```python
from build123d import *

# Parameters (mm, degrees)
SKETCH_1_R          = 32
SKETCH_1_R_2        = 24
EXTRUDE_1_DEPTH     = 2
SKETCH_2_R          = 32
SKETCH_2_R_2        = 25
EXTRUDE_2_DEPTH     = 4
SKETCH_3_R          = 1.8
CUT_EXTRUDE_1_DEPTH = 46.650848842
CUT_EXTRUDE_2_DEPTH = 2.8
SKETCH_6_R          = 1.8
CUT_EXTRUDE_3_DEPTH = 46.367830012
CUT_EXTRUDE_4_DEPTH = 2.8
FILLET_1_R          = 1


with BuildPart() as part:
    # 草图1 → 凸台-拉伸1 (new body)
    with BuildSketch(Plane.XY):
        Circle(SKETCH_1_R)
        Circle(SKETCH_1_R_2, mode=Mode.SUBTRACT)
    extrude(amount=EXTRUDE_1_DEPTH)

    # 草图2 → 凸台-拉伸2 (add)
    with BuildSketch(Plane.XY.offset(2)):
        Circle(SKETCH_2_R)
        Circle(SKETCH_2_R_2, mode=Mode.SUBTRACT)
    extrude(amount=EXTRUDE_2_DEPTH)

    # 草图3 → 切除-拉伸1 (cut, through all)
    with BuildSketch(Plane.XY.offset(6)):
        with Locations((0, 28.5)):
            Circle(SKETCH_3_R)
        with Locations((24.681724008, 14.25)):
            Circle(SKETCH_3_R)
        with Locations((24.681724008, -14.25)):
            Circle(SKETCH_3_R)
        with Locations((0, -28.5)):
            Circle(SKETCH_3_R)
        with Locations((-24.681724008, -14.25)):
            Circle(SKETCH_3_R)
        with Locations((-24.681724008, 14.25)):
            Circle(SKETCH_3_R)
    extrude(amount=-CUT_EXTRUDE_1_DEPTH, mode=Mode.SUBTRACT)

    # 草图5 → 切除-拉伸2 (cut)
    with BuildSketch(Plane.XY.offset(6)):
        Polygon((-17.866352837, 22.43873369), (-20.989347038, 23.275537464), (-23.275537464, 20.989347038), (-22.43873369, 17.866352837), (-19.31573949, 17.029549063), (-17.029549063, 19.31573949), align=None)
        Polygon((22.43873369, 17.866352837), (23.275537464, 20.989347038), (20.989347038, 23.275537464), (17.866352837, 22.43873369), (17.029549063, 19.31573949), (19.31573949, 17.029549063), align=None)
        Polygon((17.866352837, -22.43873369), (20.989347038, -23.275537464), (23.275537464, -20.989347038), (22.43873369, -17.866352837), (19.31573949, -17.029549063), (17.029549063, -19.31573949), align=None)
        Polygon((-22.43873369, -17.866352837), (-23.275537464, -20.989347038), (-20.989347038, -23.275537464), (-17.866352837, -22.43873369), (-17.029549063, -19.31573949), (-19.31573949, -17.029549063), align=None)
    extrude(amount=-CUT_EXTRUDE_2_DEPTH, mode=Mode.SUBTRACT)

    # 草图6 → 切除-拉伸3 (cut, through all)
    with BuildSketch(Plane.XY.offset(3.2)):
        with Locations((-20.152543264, 20.152543264)):
            Circle(SKETCH_6_R)
        with Locations((20.152543264, 20.152543264)):
            Circle(SKETCH_6_R)
        with Locations((20.152543264, -20.152543264)):
            Circle(SKETCH_6_R)
        with Locations((-20.152543264, -20.152543264)):
            Circle(SKETCH_6_R)
    extrude(amount=-CUT_EXTRUDE_3_DEPTH, mode=Mode.SUBTRACT)

    # 草图7 → 切除-拉伸4 (cut)
    with BuildSketch(Plane(origin=(0, 0, 0), x_dir=(-1, 0, 0), z_dir=(0, 0, -1))):
        Polygon((3.233161507, 28.5), (1.616580754, 31.3), (-1.616580754, 31.3), (-3.233161507, 28.5), (-1.616580754, 25.7), (1.616580754, 25.7), align=None)
        Polygon((26.298304762, 11.45), (27.914885515, 14.25), (26.298304762, 17.05), (23.065143254, 17.05), (21.4485625, 14.25), (23.065143254, 11.45), align=None)
        Polygon((23.065143254, -17.05), (26.298304762, -17.05), (27.914885515, -14.25), (26.298304762, -11.45), (23.065143254, -11.45), (21.4485625, -14.25), align=None)
        Polygon((-3.233161507, -28.5), (-1.616580754, -31.3), (1.616580754, -31.3), (3.233161507, -28.5), (1.616580754, -25.7), (-1.616580754, -25.7), align=None)
        Polygon((-26.298304762, -11.45), (-27.914885515, -14.25), (-26.298304762, -17.05), (-23.065143254, -17.05), (-21.4485625, -14.25), (-23.065143254, -11.45), align=None)
        Polygon((-23.065143254, 17.05), (-26.298304762, 17.05), (-27.914885515, 14.25), (-26.298304762, 11.45), (-23.065143254, 11.45), (-21.4485625, 14.25), align=None)
    extrude(amount=-CUT_EXTRUDE_4_DEPTH, mode=Mode.SUBTRACT)

    # 圆角1
    # the kernel refuses this fillet: 1 mm, written as the material it takes off along each edge
    with BuildSketch(Plane(origin=(0, 0, 6), x_dir=(1, 0, 0), z_dir=(0, -1, 0))) as fillet_1_piece_1:
        with BuildLine():
            CenterArc((25 + FILLET_1_R, -FILLET_1_R), FILLET_1_R, 90, 90)
            Line((25, -FILLET_1_R), (25, 0))
            Line((25, 0), (25 + FILLET_1_R, 0))
        make_face()
    revolve(axis=Axis((0, 0, 6), (0, 0, 1)), mode=Mode.SUBTRACT)


solid = part.part
```
Verification items for the finished model (mm, model axes). A direction names the side the tool comes from. Coordinates: 2 decimals unless noted, no trailing zeros. Loops run counter-clockwise (first coordinate to the right, second up) from the corner with the lowest first, then second, coordinate; pieces in that order, holes last. Notation, with made-up numbers: (39, -38) -> (50, -38) arc R26 cw to (50, -19) -> close; hole circle Ø10 at (78.5, 48.25). An arc over 180 degrees is marked (long way). Put each result on its own line as item: value.
1. Tool access check on faces 1 (the face through (-22, -21, 3.2)), 2 (the face through (22.246, 15.63, 1.38)), 3 (the face through (-0.234, 30.285, 4.422)). Record the directions out of +Z, -Z, +X, -X, +Y, -Y that give a thin tool (end or side, any length) a straight path to the whole face; none if there is none.
Result set:
face 1: +Z
face 2: -Z
face 3: +Z, -Z
2. Section check A-A, the plane y = 0. Record the boundary of the cut face in (x, z).
Result set:
outline: (-32, 0) -> (-24, 0) -> (-24, 2) -> (-25, 2) -> (-25, 5) arc R1 ccw to (-26, 6) -> (-32, 6) -> close; (24, 0) -> (32, 0) -> (32, 6) -> (26, 6) arc R1 ccw to (25, 5) -> (25, 2) -> (24, 2) -> close
3. Gauge pin test, flat ends, axial feed: P1, Ø4.5, axis at x = 0, y = 28.5, coming from the +Z side; P2, Ø2, axis at x = 25, y = -16, coming from the -Z side; P3, Ø1.5, axis at y = -23, z = 4, coming from the +X side; P4, Ø4, axis at x = 20.15, y = -20.15, coming from the +Z side. Record the tip position at first contact, or that the pin passes through.
Result set:
P1: stops at z = 6
P2: stops at z = 2.8
P3: stops at x = 23
P4: stops at z = 3.2
4. Section check B-B, the plane x = 0. Give the number of separate pieces and of enclosed holes in the cut face, then the cut area to 3 significant figures.
Result set:
separate pieces: 4
enclosed holes: 0
area: 33.2 mm^2
5. Thickness scan on line 1 (X direction, y = -19.5, z = 0.75); line 2 (Y direction, x = -19, z = 5.5); line 3 (Y direction, x = 0, z = 4.8). Record the ranges inside material, lowest first.
Result set:
line 1: x = -25.37 to -21.83, -18.47 to -13.99, 13.99 to 18.47, 21.83 to 25.37
line 2: y = -25.75 to -22.74, -17.35 to -16.45, 16.45 to 17.35, 22.74 to 25.75
line 3: y = -32 to -30.3, -26.7 to -25, 25 to 26.7, 30.3 to 32
